```python
from build123d import *

# Parameters (mm, degrees)
F0_W            = 25
F0_H            = 41.5
F1_DEPTH        = 30
F2_W            = 25
F2_H            = 41.5
F3_DEPTH        = 10
F4_SIZE         = 10
F6_DEPTH        = 5
F8_DEPTH        = 60.001
F10_D           = 9
F10_CBORE_D     = 15
F10_CBORE_DEPTH = 8.5


with BuildPart() as f1:
    # F0 (on Top) → F1 (new body)
    with BuildSketch(Plane.XY):
        with BuildLine():
            Line((0, -21.5), (0, 0))
            Line((0, 0), (-35, 0))
            Line((-35, 0), (-35, -41.5))
            Line((-35, -41.5), (-24.5, -41.5))
            Line((-24.5, -41.5), (-24.5, -21.5))
            ThreePointArc((-24.5, -21.5), (-20.5, -17.5), (-16.5, -21.5))
            Line((-16.5, -21.5), (0, -21.5))
        make_face()
        with Locations((-47.5, -20.75)):
            Rectangle(F0_W, F0_H)
        with BuildLine():
            Line((0, -41.5), (0, -21.5))
            Line((0, -21.5), (-16.5, -21.5))
            ThreePointArc((-16.5, -21.5), (-20.5, -17.5), (-24.5, -21.5))
            Line((-24.5, -21.5), (-24.5, -41.5))
            Line((-24.5, -41.5), (0, -41.5))
        make_face()
    extrude(amount=F1_DEPTH)

    # F2 (on face) → F3 (cut)
    with BuildSketch(Plane.XY.offset(30)):
        with Locations((-47.5, -20.75)):
            Rectangle(F2_W, F2_H)
    extrude(amount=-F3_DEPTH, mode=Mode.SUBTRACT)

    # F4
    f4_edges = [f1.edges().sort_by_distance(p)[0] for p in [
        (-60, -41.5, 10),
    ]]
    chamfer(f4_edges, length=F4_SIZE)

    # F5 (on face) → F6 (cut)
    with BuildSketch(Plane.XY.offset(30)):
        with BuildLine():
            Line((0, -21.5), (-16.5, -21.5))
            ThreePointArc((-16.5, -21.5), (-20.5, -17.5), (-24.5, -21.5))
            Line((-24.5, -21.5), (-24.5, -41.5))
            Line((-24.5, -41.5), (0, -41.5))
            Line((0, -41.5), (0, -21.5))
        make_face()
    extrude(amount=-F6_DEPTH, mode=Mode.SUBTRACT)

    # F7 (on Right) → F8 (cut, through all)
    with BuildSketch(Plane.YZ):
        Polygon((0, 0), (0, 12), (-10, 12), (-10, 11), (-21.5, 11), (-21.5, 0), align=None)
    extrude(amount=-F8_DEPTH, mode=Mode.SUBTRACT)

    # F10 (through all)
    with Locations(Plane(origin=(0, 0, 0), x_dir=(1, 0, 0), z_dir=(0, 0, -1))):
        with Locations((-15, 32)):
            CounterBoreHole(F10_D / 2, F10_CBORE_D / 2, F10_CBORE_DEPTH)

    # F11: F1 across plane


with BuildPart() as f1_1:
    add(f1.part)
    add(f1.part.mirror(Plane.YZ))

    # F12: F1 across plane


with BuildPart() as f1_2:
    add(f1_1.part)
    add(f1_1.part.mirror(Plane.XZ))


solid = f1_2.part
```
Work out the finished part from the listing and answer in its coordinate system (mm). A direction names the side the tool comes from. Give positions to 0.01 mm unless a question says otherwise; leave off trailing zeros. Order: outer loops, then holes, each group sorted by start corner. A loop starts at its lowest first (then second) coordinate and runs counter-clockwise, first axis right, second up. Notation, with made-up numbers: (66.25, -18) - (79.25, -18) arc R20 ccw to (79.25, -2) - close; hole circle Ø7 at (-36, 57). An arc over 180 degrees is marked (long way). One line per item, written item: value. Start each with the question number.
1. For a pull along X with two mould halves and no side action, classify faces 6 (the face through (-16.63, -24.68, 4.19)), 7 (the face through (-1, -16, 11)), 8 (the face through (54.9, 36.6, 9.9)), 9 (the face through (10, 32, 8.5)) as released by +X, released by -X, zero draft, split by the parting line, or undercut.
2. Section C-C, the plane x = 43.5 is taken. Write down the section's boundary in (y, z).
3. Section A-A, the plane z = 2.75 is taken. Write down the section's boundary in (x, y).
4. Section D-D, the plane z = 15.75 is taken. Write down the section's boundary in (x, y).
5. Each of these flat-tipped pins is pushed along its axis until it touches: pin 1 Ø4 at (x, y) = (-10, -14) entering from -Z; pin 2 Ø8 at (y, z) = (-33, 22.5) entering from +X; pin 3 Ø1 at (y, z) = (-19.5, 24.5) entering from -X; pin 4 Ø5.5 at (y, z) = (31, 28) entering from +X. Where does it stop, or does it pass through?
6. Consider line 1 (Y direction, x = -15, z = 5); line 2 (Y direction, x = -15, z = 18.5); line 3 (Y direction, x = 49, z = 2.5). Determine where each line is inside the solid, lowest interval first.
7. Which of the six approach directions +Z, -Z, +X, -X, +Y, -Y give full straight-line access (tool end or side, diameter ignored) to faces 1 (the face through (-1, 0, 12)), 2 (the face through (-15, 27, 8.5)), 3 (the face through (-20.4, 17.5, 27.5)), 4 (the face through (0, -32, 25)), 5 (the face through (-35, 1, 25))?
8. Section B-B, the plane y = 13.5 is taken. Write down the section's boundary in (x, z).
Filled sheet:
1. face 6: undercut
1. face 7: zero draft
1. face 8: released by +X
1. face 9: undercut
2. outline: (-41.5, 0) - (-21.5, 0) - (-21.5, 11) - (-10, 11) - (-10, 12) - (10, 12) - (10, 11) - (21.5, 11) - (21.5, 0) - (41.5, 0) - (41.5, 20) - (-41.5, 20) - close
3. outline: (-60, -31.5) - (-50, -41.5) - (50, -41.5) - (60, -31.5) - (60, -21.5) - (-60, -21.5) - close; (-60, 21.5) - (60, 21.5) - (60, 31.5) - (50, 41.5) - (-50, 41.5) - (-60, 31.5) - close; hole circle Ø15 at (-15, -32); hole circle Ø15 at (-15, 32); hole circle Ø15 at (15, -32); hole circle Ø15 at (15, 32)
4. outline: (-60, -31.5) - (-50, -41.5) - (50, -41.5) - (60, -31.5) - (60, 31.5) - (50, 41.5) - (-50, 41.5) - (-60, 31.5) - close; hole circle Ø9 at (-15, -32); hole circle Ø9 at (-15, 32); hole circle Ø9 at (15, -32); hole circle Ø9 at (15, 32)
5. pin 1: z = 11
5. pin 2: x = 60
5. pin 3: x = -35
5. pin 4: x = 35
6. line 1: -41.5 to -39.5, -24.5 to -21.5, 21.5 to 24.5, 39.5 to 41.5
6. line 2: -41.5 to -36.5, -27.5 to 27.5, 36.5 to 41.5
6. line 3: -41.5 to -21.5, 21.5 to 41.5
7. face 1: -Z, +X, -X
7. face 2: -Z
7. face 3: +Z, +Y
7. face 4: +Z, -Y
7. face 5: +Z, -X, +Y, -Y
8. outline: (-60, 11) - (60, 11) - (60, 20) - (35, 20) - (35, 30) - (-35, 30) - (-35, 20) - (-60, 20) - close
